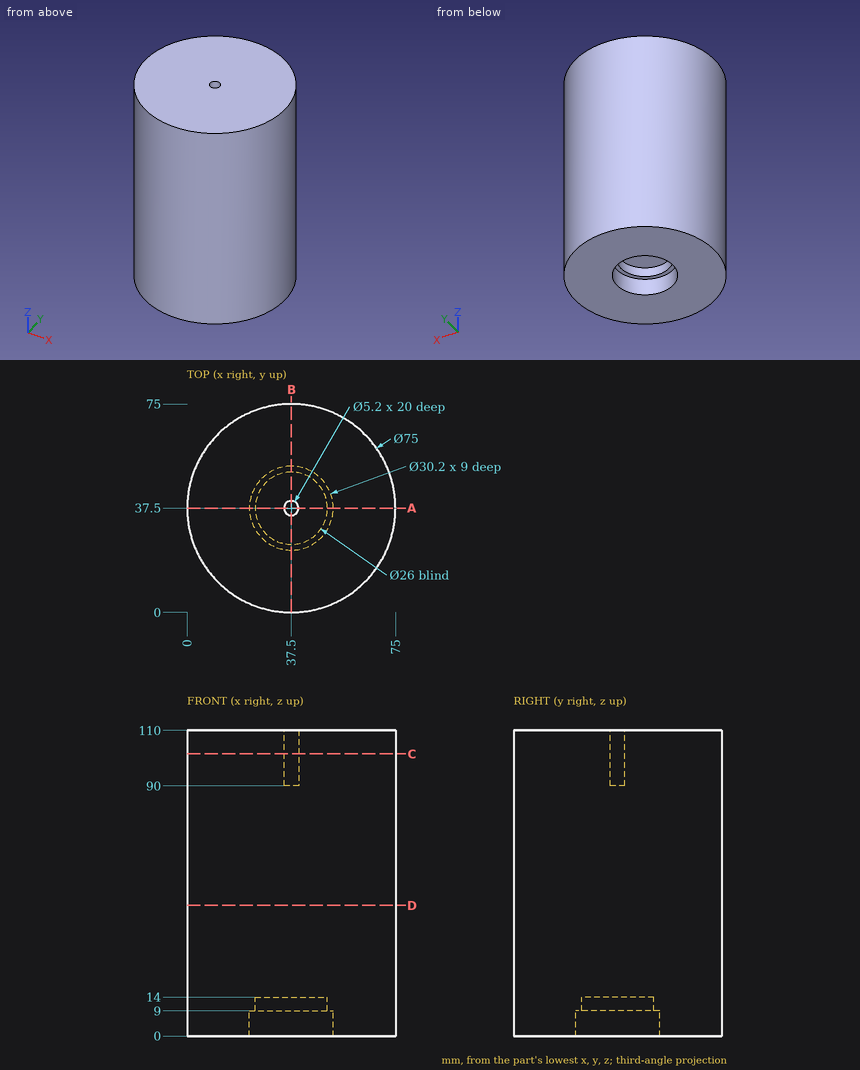
Print and shaded views of the part. All mm, measured from the part's lowest x, y and z. Give positions to 0.01 mm unless a question says otherwise; leave off trailing zeros. Write each loop counter-clockwise with the first axis right and the second up, starting at its lowest first coordinate (ties: lowest second). Pieces come first, ordered by that corner, then holes. Notation, with made-up numbers: M -29,-13 L -25,-13 A27 ccw -25,17 Z; hole C 30,5 d7. An arc over 180 degrees is marked long. Use a Markdown table: item, result.
1) Cut at D-D (z = 47). List the corners of the cut face in (x, y).
Responses:
| item | result |
|---|---|
| outline | C 37.5,37.5 d75 |
2) Drill centre lines: line 1 (Y direction, x = 37, z = 3); line 2 (Y direction, x = 37, z = 12); line 3 (Z direction, x = 45, y = 37.5). Where is each one in solid material? Low to high. Write a range as from..to.
Responses:
| item | result |
|---|---|
| line 1 | y = 0..22.41, 52.59..75 |
| line 2 | y = 0..24.51, 50.49..75 |
| line 3 | z = 14..110 |
3) Cut at A-A (y = 37.5). List the corners of the cut face in (x, z), and give its area (3 significant figures).
Responses:
| item | result |
|---|---|
| outline | M 0,0 L 22.4,0 L 22.4,9 L 24.5,9 L 24.5,14 L 50.5,14 L 50.5,9 L 52.6,9 L 52.6,0 L 75,0 L 75,110 L 40.1,110 L 40.1,90 L 34.9,90 L 34.9,110 L 0,110 Z |
| area | 7,740 mm2 |
4) Cut at C-C (z = 101.5). List the corners of the cut face in (x, y), and give its area (3 significant figures).
Responses:
| item | result |
|---|---|
| outline | C 37.5,37.5 d75; hole C 37.5,37.5 d5.2 |
| area | 4,400 mm2 |
5) Pin check, flat tips, straight feed: pin 1 (1 mm diameter, centred on x = 26, y = 34, fed in from -Z); pin 2 (1.5 mm diameter, centred on x = 26.5, z = 51, fed in from -Y); pin 3 (3 mm diameter, centred on x = 22.5, z = 39.5, fed in from +Y). Stop position of each tip, or through.
Responses:
| item | result |
|---|---|
| pin 1 | stops at z = 14 |
| pin 2 | stops at y = 1.43 |
| pin 3 | stops at y = 72.49 |
